Drawing for the job (mm, zero at the part's lowest x, y, z). A direction names the side the tool comes from. Round coordinates to 2 decimals unless told otherwise and drop trailing zeros. Write each loop counter-clockwise with the first axis right and the second up, starting at its lowest first coordinate (ties: lowest second). Pieces come first, ordered by that corner, then holes. Notation, with made-up numbers: M 46.5,10 L 102.5,10 A22 cw 102.5,24 Z; hole C -16.75,36.5 d3. An arc over 180 degrees is marked long. Use a Markdown table: item, result. Add a question column.
1) Slice it at C-C on z = 9.5. Write the cut outline in (x, y).
2) Which spindle directions (+Z, -Z, +X, -X, +Y, -Y) get a long thin tool onto all of the face, cutting with end or side? Do the marked faces 1, 2 and 3. Say none if no direction does.
3) Slice it at D-D on z = 60. Give the number of separate pieces and of enclosed holes in the cut face, plus the area to 3 significant figures.
4) Slice it at B-B on y = 14. Write the cut outline in (x, z), plus the area to 3 significant figures.
5) Slice it at A-A on x = 32. Write the cut outline in (y, z).
6) Wall check: probe 1 along Z at (x, y) = (32, 95); probe 2 along Y at (x, z) = (33, 40); probe 3 along Z at (x, y) = (33.5, 91). Give the ranges that are in metal, low to high.
7) Drop flat-ended pins along their axis: P1, Ø1.5, axis at x = 22, z = 57.5, coming from the -Y side; P2, Ø23, axis at y = 50, z = 38, coming from the +X side; P3, Ø12.5, axis at y = 12, z = 12, coming from the +X side. Give the stop position or say it passes through.
8) Two-plate mould, pull along Z, no slides. Class the marked faces 4, 5 and 6: released by +Z, released by -Z, zero draft, split by the parting line, or undercut.
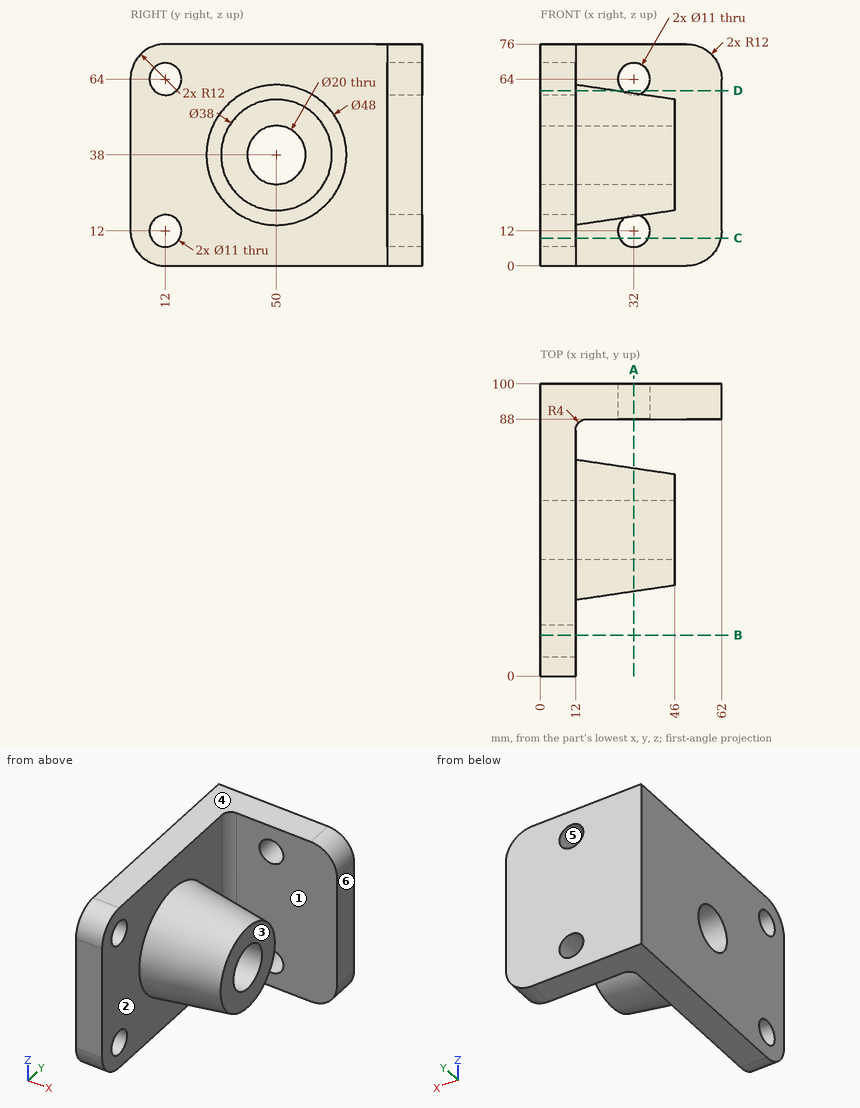
Entries:
| question | item | result |
|---|---|---|
| 1 | outline | M 0,0.26 L 12,0.26 L 12,7.1 L 0,7.1 Z; M 0,16.9 L 12,16.9 L 12,84 A4 cw 16,88 L 27.1,88 L 27.1,100 L 0,100 Z; M 36.9,88 L 61.74,88 L 61.74,100 L 36.9,100 Z |
| 2 | face 1 | +Z, -Z, +X |
| 2 | face 2 | +X |
| 2 | face 3 | +Z, -Z, +X, -Y |
| 3 | separate pieces | 3 |
| 3 | enclosed holes | 0 |
| 3 | area | 1,790 mm^2 |
| 4 | outline | M 0,0 L 12,0 L 12,6.88 L 0,6.88 Z; M 0,17.12 L 12,17.12 L 12,58.88 L 0,58.88 Z; M 0,69.12 L 12,69.12 L 12,76 L 0,76 Z |
| 4 | area | 666 mm^2 |
| 5 | outline | C 50,38 d42.12; M 88,0 L 100,0 L 100,6.5 L 88,6.5 Z; M 88,17.5 L 100,17.5 L 100,58.5 L 88,58.5 Z; M 88,69.5 L 100,69.5 L 100,76 L 88,76 Z; hole C 50,38 d20 |
| 6 | probe 1 | z = 0 to 6.5, 17.5 to 58.5, 69.5 to 76 |
| 6 | probe 2 | y = 29.18 to 40.2, 59.8 to 70.82, 88 to 100 |
| 6 | probe 3 | z = 0 to 6.71, 17.29 to 58.71, 69.29 to 76 |
| 7 | P1 | stops at y = 37.49 |
| 7 | P2 | stops at x = 46 |
| 7 | P3 | stops at x = 12 |
| 8 | face 4 | released by +Z |
| 8 | face 5 | undercut |
| 8 | face 6 | zero draft |
